from build123d import *

# Parameters (mm, degrees)
F0_R     = 20
F0_R_2   = 13
F3_R     = 39
F3_R_2   = 20
F3_R_3   = 13
F4_DEPTH = 8
F5_R     = 5
F5_R_2   = 13
F6_DEPTH = 11


with BuildPart() as f2:
    # F2: sweep along a path in F1
    with BuildLine(Plane.XZ) as f2_path:
        Line((0, 0), (0, 23))
        ThreePointArc((0, 23), (-10.2512626585, 47.7487373415), (-35, 58))
        Line((-35, 58), (-88, 58))
    # F0 (on Top) → F2 (sweep)
    with BuildSketch(Plane.XY):
        Circle(F0_R)
        Circle(F0_R_2, mode=Mode.SUBTRACT)
    sweep(path=f2_path.line)

    # F3 (on face) → F4 (join)
    with BuildSketch(Plane(origin=(-88, 0, 0), x_dir=(0, -1, 0), z_dir=(-1, 0, 0))):
        with Locations((0, 58)):
            Circle(F3_R)
        with BuildLine():
            ThreePointArc((4.982608643, 87.5833333333), (21.2132034356, 79.2132034356), (29.5833333333, 62.982608643))
            ThreePointArc((29.5833333333, 62.982608643), (33.3850160019, 61.679900361), (35, 58))
            ThreePointArc((35, 58), (33.3850160019, 54.320099639), (29.5833333333, 53.017391357))
            ThreePointArc((29.5833333333, 53.017391357), (21.2132034356, 36.7867965644), (4.982608643, 28.4166666667))
            ThreePointArc((4.982608643, 28.4166666667), (4.9956502687, 28.2085147299), (5, 28))
            ThreePointArc((5, 28), (-0.2085147299, 23.0043497313), (-4.982608643, 28.4166666667))
            ThreePointArc((-4.982608643, 28.4166666667), (-21.2132034356, 36.7867965644), (-29.5833333333, 53.017391357))
            ThreePointArc((-29.5833333333, 53.017391357), (-35, 58), (-29.5833333333, 62.982608643))
            ThreePointArc((-29.5833333333, 62.982608643), (-21.2132034356, 79.2132034356), (-4.982608643, 87.5833333333))
            ThreePointArc((-4.982608643, 87.5833333333), (-0.2085147299, 92.9956502687), (5, 88))
            ThreePointArc((5, 88), (4.9956502687, 87.7914852701), (4.982608643, 87.5833333333))
        make_face(mode=Mode.SUBTRACT)
        with BuildLine():
            ThreePointArc((29.5833333333, 53.017391357), (25, 58), (29.5833333333, 62.982608643))
            ThreePointArc((29.5833333333, 62.982608643), (21.2132034356, 79.2132034356), (4.982608643, 87.5833333333))
            ThreePointArc((4.982608643, 87.5833333333), (0, 83), (-4.982608643, 87.5833333333))
            ThreePointArc((-4.982608643, 87.5833333333), (-21.2132034356, 79.2132034356), (-29.5833333333, 62.982608643))
            ThreePointArc((-29.5833333333, 62.982608643), (-26.320099639, 61.3850160019), (-25, 58))
            ThreePointArc((-25, 58), (-26.320099639, 54.6149839981), (-29.5833333333, 53.017391357))
            ThreePointArc((-29.5833333333, 53.017391357), (-21.2132034356, 36.7867965644), (-4.982608643, 28.4166666667))
            ThreePointArc((-4.982608643, 28.4166666667), (0, 33), (4.982608643, 28.4166666667))
            ThreePointArc((4.982608643, 28.4166666667), (21.2132034356, 36.7867965644), (29.5833333333, 53.017391357))
        make_face()
        with Locations((0, 58)):
            Circle(F3_R_2, mode=Mode.SUBTRACT)
        with Locations((0, 58)):
            Circle(F3_R_2)
        with Locations((0, 58)):
            Circle(F3_R_3, mode=Mode.SUBTRACT)
    extrude(amount=-F4_DEPTH)

    # F5 (on Top) → F6 (join)
    with BuildSketch(Plane.XY):
        with BuildLine():
            Line((22.3639873232, 26.9230769231), (9.5845659957, 37.5384615385))
            ThreePointArc((9.5845659957, 37.5384615385), (0, 41), (-9.5845659957, 37.5384615385))
            Line((-9.5845659957, 37.5384615385), (-22.3639873232, 26.9230769231))
            ThreePointArc((-22.3639873232, 26.9230769231), (-35, 0), (-22.3639873232, -26.9230769231))
            Line((-22.3639873232, -26.9230769231), (-9.5845659957, -37.5384615385))
            ThreePointArc((-9.5845659957, -37.5384615385), (0, -41), (9.5845659957, -37.5384615385))
            Line((9.5845659957, -37.5384615385), (22.3639873232, -26.9230769231))
            ThreePointArc((22.3639873232, -26.9230769231), (35, 0), (22.3639873232, 26.9230769231))
        make_face()
        with Locations((0, -26)):
            Circle(F5_R, mode=Mode.SUBTRACT)
        Circle(F5_R_2, mode=Mode.SUBTRACT)
        with Locations((0, 26)):
            Circle(F5_R, mode=Mode.SUBTRACT)
    extrude(amount=F6_DEPTH)


solid = f2.part
Geometry check sheet. Reference: the model listing, model coordinates, mm. A direction names the side the tool comes from. Coordinates: 2 decimals unless noted, no trailing zeros. Order: outer loops, then holes, each group sorted by start corner. A loop starts at its lowest first (then second) coordinate and runs counter-clockwise, first axis right, second up. Notation, with made-up numbers: (54, 56) - (112, 56) arc R7 cw to (112, 63) - close; hole circle Ø2 at (21, 47.25). An arc over 180 degrees is marked (long way). Answer in a Markdown table with one row per item. Add a question column.
1) Set-up check for faces 4 (the cylindrical face through (-57.815, 6.007, 77.076)), 5 (the cylindrical face through (-10.316, -7.91, 11.661)), 6 (the cylindrical face through (-35, 0, 5)): record each of +Z, -Z, +X, -X, +Y, -Y from which the full face is reachable in a straight line by a thin tool's end or side.
2) Gauge pin test, flat ends, axial feed: P1, Ø9, axis at x = 0, y = 26, coming from the +Z side; P2, Ø10, axis at x = -18, z = 51, coming from the +Y side; P3, Ø3, axis at x = -41.5, y = -2.5, coming from the +Z side (3 decimals); P4, Ø12, axis at x = 21, y = 21, coming from the +Z side. Record the tip position at first contact, or that the pin passes through.
3) Cross-section at D-D, the plane x = 0. State how many separate pieces and enclosed holes the cut face has, then the cut area to 3 significant figures.
4) Cross-section at C-C, the plane x = -47. Record the cut outline in (y, z), then the cut area to 3 significant figures.
5) Release check for a two-part mould opening along Y. For faces 1 (the cylindrical face through (-1.08, -30.88, 5.42)), 2 (the flat face through (-80, -17, 41)), 3 (the cylindrical face through (-84.056, 8.454, 19.927)) record: +Y half, -Y half, draft (parallel to the pull), parting line (faces both ways), or undercut.
6) Cross-section at A-A, the plane z = 7.5. Record the cut outline in (x, y), then the cut area to 3 significant figures.
7) Material ranges on line 1 along Y through (x, z) = (0, 5.75); line 2 along X through (y, z) = (6, 33.5); line 3 along Y through (x, z) = (0, 12.75), recorded low to high. Write a range as [from, to].
8) Cross-section at B-B, the plane y = -8. Record the cut outline in (x, z), then the cut area to 3 significant figures.
Check result:
| question | item | result |
|---|---|---|
| 1 | face 4 | none |
| 1 | face 5 | -Z |
| 1 | face 6 | -Z, -X |
| 2 | P1 | passes through |
| 2 | P2 | stops at y = 20 |
| 2 | P3 | stops at z = 77.975 |
| 2 | P4 | stops at z = 11 |
| 3 | separate pieces | 3 |
| 3 | enclosed holes | 0 |
| 3 | area | 1,280 mm² |
| 4 | outline | circle Ø40 at (0, 58); hole circle Ø26 at (0, 58) |
| 4 | area | 726 mm² |
| 5 | face 1 | undercut |
| 5 | face 2 | draft |
| 5 | face 3 | parting line |
| 6 | outline | (-22.36, -26.92) - (-9.58, -37.54) arc R15 ccw to (9.58, -37.54) - (22.36, -26.92) arc R35 ccw to (22.36, 26.92) - (9.58, 37.54) arc R15 ccw to (-9.58, 37.54) - (-22.36, 26.92) arc R35 ccw to start; hole circle Ø26 at (0, 0); hole circle Ø10 at (0, -26); hole circle Ø10 at (0, 26) |
| 6 | area | 3,440 mm² |
| 7 | line 1 | y = [-41, -31], [-21, -13], [13, 21], [31, 41] |
| 7 | line 2 | x = [-88, -80], [-23.03, -14.01], [10.33, 18.05] |
| 7 | line 3 | y = [-20, -13], [13, 20] |
| 8 | outline | (-88, 19.83) - (-80, 19.83) - (-80, 39.67) - (-35, 39.67) arc R16.67 cw to (-18.33, 23) - (-18.33, 11) - (-34.07, 11) - (-34.07, 0) - (-10.25, 0) - (-10.25, 23) arc R24.75 ccw to (-35, 47.75) - (-88, 47.75) - close; (-88, 68.25) - (-35, 68.25) arc R45.25 cw to (10.25, 23) - (10.25, 0) - (34.07, 0) - (34.07, 11) - (18.33, 11) - (18.33, 23) arc R53.33 ccw to (-35, 76.33) - (-80, 76.33) - (-80, 96.17) - (-88, 96.17) - close |
| 8 | area | 2,780 mm² |
